```python
from build123d import *

# Parameters (mm, degrees)
F0_R     = 15
F1_DEPTH = 30
F3_D     = 22.4
F3_DEPTH = 12
F3_TIP   = 6.7296389331
F4_SIZE2 = 2
F4_SIZE  = 3


with BuildPart() as f1:
    # F0 (on Top) → F1 (new body)
    with BuildSketch(Plane.XY):
        Circle(F0_R)
    extrude(amount=F1_DEPTH)

    # F3
    with Locations(Plane(origin=(0, 0, 0), x_dir=(1, 0, 0), z_dir=(0, 0, -1))):
        with Locations((0, 0)):
            Hole(F3_D / 2, depth=F3_DEPTH)
            with Locations((0, 0, -(F3_DEPTH + F3_TIP / 2))):  # 118° drill point
                Cone(0, F3_D / 2, F3_TIP, mode=Mode.SUBTRACT)

    # F4
    f4_edges = [f1.edges().sort_by_distance(p)[0] for p in [
        (-15, 0, 0),
    ]]
    f4_side = f1.faces().sort_by_distance((-15, 0, 15))[0]
    chamfer(f4_edges, length=F4_SIZE, length2=F4_SIZE2, reference=f4_side)


solid = f1.part
```
For this review, take the finished solid that the model builds, in its own axes (mm). Round coordinates to 2 decimals unless told otherwise and drop trailing zeros. Write each loop counter-clockwise with the first axis right and the second up, starting at its lowest first coordinate (ties: lowest second). Pieces come first, ordered by that corner, then holes. Notation, with made-up numbers: M 26.25,39 L 67.25,39 A34 ccw 67.25,77 Z; hole C -30.5,72.25 d10. An arc over 180 degrees is marked long. One line per item, written item: value. Start each with the question number.
(1) Insertion check: pin 1 (18 mm diameter, centred on x = 0, y = 0, fed in from -Z); pin 2 (4 mm diameter, centred on x = 6.5, z = 14, fed in from -Y); pin 3 (2 mm diameter, centred on x = 2.5, z = 5, fed in from +Y). Each pin has a flat end and moves straight along its axis. Give the tip position at first contact, or say it passes through.
(2) The part is to be moulded in two halves that separate along Y. For faces 1 (the cylindrical face through (-14.985, 0.66, 16.311)), 2 (the flat face through (0, 0, 30)), 3 (the conical face through (1.05, -1.64, 17.56)), 4 (the cylindrical face through (11.19, -0.49, 6.08)), say which applies: released by +Y, released by -Y, zero draft, split by the parting line, or undercut.
(3) We need section A-A (z = 5). Give the boundary of the cut face in (x, y), and give its area (3 significant figures).
(4) We need section B-B (z = 26.5). Give the boundary of the cut face in (x, y).
(5) Wall thickness on line 1 (Y direction, x = 0, z = 7); line 2 (Y direction, x = -2.5, z = 8.25); line 3 (X direction, y = -7.5, z = 12.5): over which ranges is each line inside the solid? List them lowest first.
(6) We need section C-C (z = 15.75). Give the boundary of the cut face in (x, y).
Result:
1. pin 1: z = 13.32
1. pin 2: y = -14.31
1. pin 3: y = 14.92
2. face 1: split by the parting line
2. face 2: zero draft
2. face 3: undercut
2. face 4: undercut
3. outline: C 0,0 d30; hole C 0,0 d22.4
3. area: 313 mm²
4. outline: C 0,0 d30
5. line 1: -15 to -11.2, 11.2 to 15
5. line 2: -14.79 to -10.92, 10.92 to 14.79
5. line 3: -12.99 to -7.16, 7.16 to 12.99
6. outline: C 0,0 d30; hole C 0,0 d9.92
